Design review of the part built by this model. Coordinates are the model's own, in mm. Face numbers are marked on the shaded views. A direction names the side the tool comes from. Coordinates: 2 decimals unless noted, no trailing zeros. Loops run counter-clockwise (first coordinate to the right, second up) from the corner with the lowest first, then second, coordinate; pieces in that order, holes last.
Q1. Add section A-A on z = -67.5. Give the boundary of the cut face in (x, y) (3 decimals).
Q2. Wall thickness on probe 1 along X at (y, z) = (1.05, -67.5); probe 2 along Z at (x, y) = (-110, 2.7); probe 3 along X at (y, z) = (6, 0): over which ranges is each line inside the solid? List them lowest first.
Q3. Machinability: for the marked faces 1, 2, 3, 4 and 5, which of the approach directions +Z, -Z, +X, -X, +Y, -Y give a long, thin tool a straight path to every point of the face, cutting with its end or side? Answer none if there is none.
Q4. Add section C-C on y = 79. Give the boundary of the cut face in (x, z), and give its area (3 significant figures).
Q5. Add section B-B on x = -76. Give the boundary of the cut face in (y, z), and give its area (3 significant figures).
Q6. Add section D-D on z = -42. Give the boundary of the cut face in (x, y).
Q7. Draft analysis for pull direction X (two halves, no side actions). For the marked faces 6, 7, 8 and 9, state which applies: released by +X, released by -X, zero draft, split by the parting line, or undercut.
Q8. For P1, Ø5, axis at y = 19.5, z = 70, coming from the -X side; P2, Ø3, axis at y = 30, z = -65.5, coming from the -X side; P3, Ø4.5, axis at x = -113, z = -70.5, coming from the +Y side, all flat-tipped, find the tip position at first contact; note any pin that passes through.
```python
from build123d import *

# Parameters (mm, degrees)
SZKIC1_W                        = 200
SZKIC1_H                        = 200
DODANIE_WYCI_GNI_CIE1_DEPTH     = 30
WYTNIJ_WYCI_GNI_CIE1_DEPTH      = 145.568322948
WYTNIJ_WYCI_GNI_CIE1_DEPTH_BACK = 145.568322948
SZKIC2_W                        = 80
SZKIC2_H                        = 16
WYTNIJ_WYCI_GNI_CIE2_DEPTH      = 145.568322948
WYTNIJ_WYCI_GNI_CIE2_DEPTH_BACK = 145.568322948
SZKIC3_R                        = 20
SZKIC4_W                        = 28
SZKIC4_H                        = 16
DODANIE_WYCI_GNI_CIE2_DEPTH     = 9
DODANIE_WYCI_GNI_CIE3_START     = 30
SZKIC5_W                        = 50
SZKIC5_H                        = 50
DODANIE_WYCI_GNI_CIE3_DEPTH     = 40
DODANIE_WYCI_GNI_CIE4_START     = 70
SZKIC6_W                        = 151.215135745
SZKIC6_H                        = 50
SZKIC6_R                        = 9.5
DODANIE_WYCI_GNI_CIE4_DEPTH     = 5
DODANIE_WYCI_GNI_CIE5_START     = 75
SZKIC7_W                        = 151.215135745
SZKIC7_H                        = 50
SZKIC7_R                        = 15
DODANIE_WYCI_GNI_CIE5_DEPTH     = 15
DODANIE_WYCI_GNI_CIE6_START     = 60
DODANIE_WYCI_GNI_CIE6_DEPTH     = 25
WYTNIJ_WYCI_GNI_CIE3_DEPTH      = 181.277563773
WYTNIJ_WYCI_GNI_CIE4_START      = 5
WYTNIJ_WYCI_GNI_CIE4_DEPTH      = 176.277563773
SZYK_LINIOWY1_OUTLINE_R         = 7.5
SZYK_LINIOWY1_OUTLINE_R_2       = 2.75
SZYK_LINIOWY1_DEPTH             = 5
SZYK_LINIOWY1_2_OUTLINE_W       = 20
SZYK_LINIOWY1_2_OUTLINE_H       = 25
SZYK_LINIOWY1_2_OUTLINE_R       = 7.5
SZYK_LINIOWY1_2_DEPTH           = 30
SZYK_START                      = -113
SZYK_LINIOWY1_3_OUTLINE_W       = 35
SZYK_LINIOWY1_3_OUTLINE_H       = 25
SZYK_LINIOWY1_3_DEPTH           = 16.172267629
ZAOKR_GLENIE1_R                 = 20
SFAZOWANIE1_SIZE                = 10
SZKIC10_R                       = 2.6
WYTNIJ_WYCI_GNI_CIE5_DEPTH      = 176.957381204
WYTNIJ_WYCI_GNI_CIE6_DEPTH      = 181.277563773
WYTNIJ_WYCI_GNI_CIE6_DEPTH_BACK = 5
SZKIC11_R                       = 6


with BuildPart() as part:
    # Szkic1 → Dodanie-wyciągnięcie1 (new body)
    with BuildSketch(Plane(origin=(0, 0, 0), x_dir=(1, 0, 0), z_dir=(0, 1, 0))):
        Rectangle(SZKIC1_W, SZKIC1_H)
    extrude(amount=DODANIE_WYCI_GNI_CIE1_DEPTH)

    # Szkic2 → Wytnij-wyciągnięcie1 (cut, two sides: drawn at the far end of the back side and taken through both)
    with BuildSketch(Plane(origin=(0, 0, 0), x_dir=(1, 0, 0), z_dir=(0, 1, 0)).offset(-WYTNIJ_WYCI_GNI_CIE1_DEPTH_BACK)):
        Rectangle(SZKIC2_W, SZKIC2_H)
    extrude(amount=WYTNIJ_WYCI_GNI_CIE1_DEPTH + WYTNIJ_WYCI_GNI_CIE1_DEPTH_BACK, mode=Mode.SUBTRACT)

    # Szkic3 → Wytnij-wyciągnięcie2 (cut, two sides: drawn at the far end of the back side and taken through both)
    with BuildSketch(Plane(origin=(0, 0, 0), x_dir=(1, 0, 0), z_dir=(0, 1, 0)).offset(-WYTNIJ_WYCI_GNI_CIE2_DEPTH_BACK)):
        with Locations((33.228865647, 0)):
            Circle(SZKIC3_R)
    extrude(amount=WYTNIJ_WYCI_GNI_CIE2_DEPTH + WYTNIJ_WYCI_GNI_CIE2_DEPTH_BACK, mode=Mode.SUBTRACT)

    # Szkic4 → Dodanie-wyciągnięcie2 (add)
    with BuildSketch(Plane(origin=(0, 0, 0), x_dir=(1, 0, 0), z_dir=(0, 1, 0))):
        with Locations((-26, 0)):
            Rectangle(SZKIC4_W, SZKIC4_H)
    extrude(amount=DODANIE_WYCI_GNI_CIE2_DEPTH)

    # Szkic5 → Dodanie-wyciągnięcie3 (add)
    with BuildSketch(Plane(origin=(0, 0, 0), x_dir=(1, 0, 0), z_dir=(0, 1, 0)).offset(DODANIE_WYCI_GNI_CIE3_START)):
        with Locations((-70, 0)):
            Rectangle(SZKIC5_W, SZKIC5_H)
    extrude(amount=DODANIE_WYCI_GNI_CIE3_DEPTH)

    # Szkic6 → Dodanie-wyciągnięcie4 (add)
    with BuildSketch(Plane(origin=(0, 0, 0), x_dir=(1, 0, 0), z_dir=(0, 1, 0)).offset(DODANIE_WYCI_GNI_CIE4_START)):
        with Locations((-19.392432127, 0)):
            Rectangle(SZKIC6_W, SZKIC6_H)
        with Locations(Location((33.228865647, 0, 0), (0, 0, 90))):
            Circle(SZKIC6_R, mode=Mode.SUBTRACT)
    extrude(amount=DODANIE_WYCI_GNI_CIE4_DEPTH)

    # Szkic7 → Dodanie-wyciągnięcie5 (add)
    with BuildSketch(Plane(origin=(0, 0, 0), x_dir=(1, 0, 0), z_dir=(0, 1, 0)).offset(DODANIE_WYCI_GNI_CIE5_START)):
        with Locations((-19.392432127, 0)):
            Rectangle(SZKIC7_W, SZKIC7_H)
        with Locations(Location((33.228865647, 0, 0), (0, 0, 270))):
            Circle(SZKIC7_R, mode=Mode.SUBTRACT)
    extrude(amount=DODANIE_WYCI_GNI_CIE5_DEPTH)

    # Szkic8 → Dodanie-wyciągnięcie6 (add)
    with BuildSketch(Plane.XY.offset(DODANIE_WYCI_GNI_CIE6_START)):
        Polygon((-100, 0), (-120, 0), (-120, 5), (-100, 30), align=None)
    dodanie_wyci_gni_cie6 = extrude(amount=DODANIE_WYCI_GNI_CIE6_DEPTH)

    # Szkic9 → Wytnij-wyciągnięcie3 (cut, symmetric)
    with BuildSketch(Plane(origin=(0, 0, 0), x_dir=(1, 0, 0), z_dir=(0, 1, 0))):
        with BuildLine():
            ThreePointArc((-107.25, -72.5), (-107.5214161, -71.308730991), (-108.282088619, -70.352610774))
            Line((-108.282088619, -70.352610774), (-111.717911381, -74.647389226))
            ThreePointArc((-111.717911381, -74.647389226), (-108.808730991, -74.9785839), (-107.25, -72.5))
        make_face()
        with BuildLine():
            Line((-111.717911381, -74.647389226), (-108.282088619, -70.352610774))
            ThreePointArc((-108.282088619, -70.352610774), (-112.147389226, -70.782088619), (-111.717911381, -74.647389226))
        make_face()
    wytnij_wyci_gni_cie3 = extrude(amount=WYTNIJ_WYCI_GNI_CIE3_DEPTH, both=True, mode=Mode.SUBTRACT)

    # Szkic9<3> → Wytnij-wyciągnięcie4 (cut, through all)
    with BuildSketch(Plane(origin=(0, 0, 0), x_dir=(1, 0, 0), z_dir=(0, 1, 0)).offset(WYTNIJ_WYCI_GNI_CIE4_START)):
        with BuildLine():
            ThreePointArc((-102.5, -72.5), (-103.240225728, -69.251084521), (-105.314787143, -66.643483929))
            Line((-105.314787143, -66.643483929), (-108.282088619, -70.352610774))
            ThreePointArc((-108.282088619, -70.352610774), (-107.5214161, -71.308730991), (-107.25, -72.5))
            ThreePointArc((-107.25, -72.5), (-108.808730991, -74.9785839), (-111.717911381, -74.647389226))
            Line((-111.717911381, -74.647389226), (-114.685212857, -78.356516071))
            ThreePointArc((-114.685212857, -78.356516071), (-106.751084521, -79.259774272), (-102.5, -72.5))
        make_face()
        with BuildLine():
            Line((-108.282088619, -70.352610774), (-105.314787143, -66.643483929))
            ThreePointArc((-105.314787143, -66.643483929), (-115.856516071, -67.814787143), (-114.685212857, -78.356516071))
            Line((-114.685212857, -78.356516071), (-111.717911381, -74.647389226))
            ThreePointArc((-111.717911381, -74.647389226), (-112.147389226, -70.782088619), (-108.282088619, -70.352610774))
        make_face()
    wytnij_wyci_gni_cie4 = extrude(amount=WYTNIJ_WYCI_GNI_CIE4_DEPTH, mode=Mode.SUBTRACT)



with BuildPart() as body_2:
    # Szyk liniowy1: read off the stored shape, not the designer's step
    # Szyk liniowy1 outline → Szyk liniowy1 (new body)
    with BuildSketch(Plane(origin=(0, 0, 0), x_dir=(1, 0, 0), z_dir=(0, 1, 0))):
        with Locations((-110, 67.5)):
            Circle(SZYK_LINIOWY1_OUTLINE_R)
        with Locations((-110, 67.5)):
            Circle(SZYK_LINIOWY1_OUTLINE_R_2, mode=Mode.SUBTRACT)
    szyk_liniowy1 = extrude(amount=SZYK_LINIOWY1_DEPTH)


with BuildPart() as part_1:
    add(part.part)

    add(body_2.part)  # Szyk liniowy1 2 merges body 2
    # Szyk liniowy1 2 outline → Szyk liniowy1 2 (add)
    with BuildSketch(Plane(origin=(0, 0, 0), x_dir=(1, 0, 0), z_dir=(0, 1, 0))):
        with Locations((-110, 67.5)):
            Rectangle(SZYK_LINIOWY1_2_OUTLINE_W, SZYK_LINIOWY1_2_OUTLINE_H)
        with Locations((-110, 67.5)):
            Circle(SZYK_LINIOWY1_2_OUTLINE_R, mode=Mode.SUBTRACT)
    szyk_liniowy1_2 = extrude(amount=SZYK_LINIOWY1_2_DEPTH)

    # Szyk liniowy1 3 outline → Szyk liniowy1 3 (cut)
    with BuildSketch(Plane(origin=(0, 0, 0), x_dir=(0.6246950475544242, 0.7808688094430304, 0), z_dir=(0.7808688094430304, -0.6246950475544242, 0)).offset(SZYK_START)):
        with Locations((-55.5, -67.5)):
            Rectangle(SZYK_LINIOWY1_3_OUTLINE_W, SZYK_LINIOWY1_3_OUTLINE_H)
    szyk_liniowy1_3 = extrude(amount=SZYK_LINIOWY1_3_DEPTH, mode=Mode.SUBTRACT)

    # Lustro1: Dodanie-wyciągnięcie6, Wytnij-wyciągnięcie3, Wytnij-wyciągnięcie4, Szyk liniowy1, Szyk liniowy1 2, Szyk liniowy1 3 across plane
    add(dodanie_wyci_gni_cie6.mirror(Plane(origin=(0, 0, 0), x_dir=(0, 0, 1), z_dir=(1, 0, 0))))
    add(wytnij_wyci_gni_cie3.mirror(Plane(origin=(0, 0, 0), x_dir=(0, 0, 1), z_dir=(1, 0, 0))), mode=Mode.SUBTRACT)
    add(wytnij_wyci_gni_cie4.mirror(Plane(origin=(0, 0, 0), x_dir=(0, 0, 1), z_dir=(1, 0, 0))), mode=Mode.SUBTRACT)
    add(szyk_liniowy1.mirror(Plane(origin=(0, 0, 0), x_dir=(0, 0, 1), z_dir=(1, 0, 0))))
    add(szyk_liniowy1_2.mirror(Plane(origin=(0, 0, 0), x_dir=(0, 0, 1), z_dir=(1, 0, 0))))
    add(szyk_liniowy1_3.mirror(Plane(origin=(0, 0, 0), x_dir=(0, 0, 1), z_dir=(1, 0, 0))), mode=Mode.SUBTRACT)

    # Zaokrąglenie1
    # the kernel refuses this fillet: 20 mm, written as the material it takes off along each edge
    with BuildSketch(Plane(origin=(-100, -48.412291828, 100), x_dir=(1, 0, 0), z_dir=(0, 1, 0))) as zaokr_glenie1_piece_1:
        with BuildLine():
            CenterArc((19.364916731, 20), ZAOKR_GLENIE1_R, 194.477512186, 75.522487814)
            Line((0, 15), (-0.387298335, 14.9))
            ThreePointArc((-0.387298335, 14.9), (-0.4, 7.5), (-0.4, 0))
            Line((-0.4, 0), (0, -0.4))
            Line((0, -0.4), (19.364916731, -0.4))
            Line((19.364916731, -0.4), (19.364916731, 0))
        make_face()
    extrude(amount=126.824583655, mode=Mode.SUBTRACT)
    with BuildSketch(Plane(origin=(-100, -50, -100), x_dir=(0, 0, 1), z_dir=(0, 1, 0)), Plane(origin=(100, -50, -100), x_dir=(-1, 0, 0), z_dir=(0, 1, 0))) as zaokr_glenie1_piece_2:
        with BuildLine():
            CenterArc((ZAOKR_GLENIE1_R, ZAOKR_GLENIE1_R), ZAOKR_GLENIE1_R, 180, 90)
            Line((0, ZAOKR_GLENIE1_R), (-ZAOKR_GLENIE1_R * 0.02, ZAOKR_GLENIE1_R))
            Line((-ZAOKR_GLENIE1_R * 0.02, ZAOKR_GLENIE1_R), (-ZAOKR_GLENIE1_R * 0.02, -ZAOKR_GLENIE1_R * 0.02))
            Line((-ZAOKR_GLENIE1_R * 0.02, -ZAOKR_GLENIE1_R * 0.02), (ZAOKR_GLENIE1_R, -ZAOKR_GLENIE1_R * 0.02))
            Line((ZAOKR_GLENIE1_R, -ZAOKR_GLENIE1_R * 0.02), (ZAOKR_GLENIE1_R, 0))
        make_face()
    extrude(amount=130, mode=Mode.SUBTRACT)
    with BuildSketch(Plane(origin=(100, -48.412291828, 100), x_dir=(-1, 0, 0), z_dir=(0, 1, 0))) as zaokr_glenie1_piece_3:
        with BuildLine():
            CenterArc((19.364916731, -20), ZAOKR_GLENIE1_R, 90, 75.522487814)
            Line((0, -15), (-0.387298335, -14.9))
            ThreePointArc((-0.387298335, -14.9), (-0.4, -7.5), (-0.4, 0))
            Line((-0.4, 0), (0, 0.4))
            Line((0, 0.4), (19.364916731, 0.4))
            Line((19.364916731, 0.4), (19.364916731, 0))
        make_face()
    extrude(amount=126.824583655, mode=Mode.SUBTRACT)

    # Sfazowanie1
    sfazowanie1_edges = [part_1.edges().sort_by_distance(p)[0] for p in [
        (-45, 70, 0),
    ]]
    chamfer(sfazowanie1_edges, length=SFAZOWANIE1_SIZE)

    # Szkic10 → Wytnij-wyciągnięcie5 (cut, through all)
    with BuildSketch(Plane(origin=(0, 9, 0), x_dir=(1, 0, 0), z_dir=(0, 1, 0))):
        with Locations(Location((-35, 0, 0), (0, 0, 270))):
            Circle(SZKIC10_R)
        with Locations(Location((-20, 0, 0), (0, 0, 270))):
            Circle(SZKIC10_R)
    extrude(amount=-WYTNIJ_WYCI_GNI_CIE5_DEPTH, mode=Mode.SUBTRACT)

    # Szkic11 → Wytnij-wyciągnięcie6 (cut, two sides: drawn at the far end of the back side and taken through both)
    with BuildSketch(Plane(origin=(0, 0, 0), x_dir=(-1, 0, 0), z_dir=(0, -1, 0)).offset(-WYTNIJ_WYCI_GNI_CIE6_DEPTH_BACK)):
        with Locations(Location((20, 0, 0), (0, 0, 270))):
            Circle(SZKIC11_R)
        with Locations(Location((35, 0, 0), (0, 0, 270))):
            Circle(SZKIC11_R)
    extrude(amount=WYTNIJ_WYCI_GNI_CIE6_DEPTH + WYTNIJ_WYCI_GNI_CIE6_DEPTH_BACK, mode=Mode.SUBTRACT)


solid = part_1.part
```
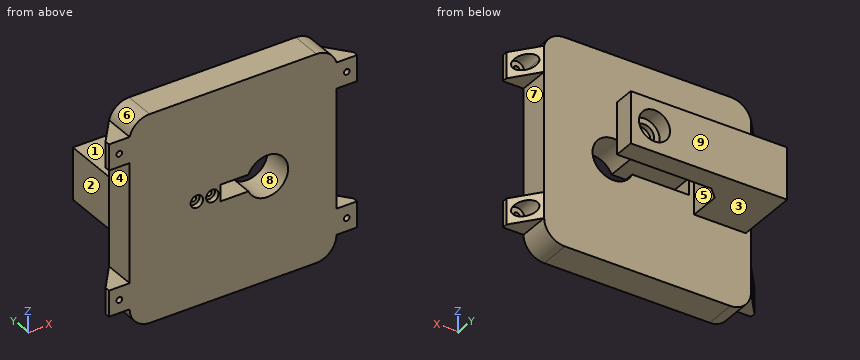
Entries:
1. outline: (-120, 0) - (-112.75, 0) - (-112.75, 5) - (-117.5, 5) - (-117.5, 8.125) - (-120, 5) - close; (-107.25, 0) - (107.25, 0) - (107.25, 5) - (102.5, 5) - (102.5, 26.875) - (100, 30) - (-100, 30) - (-102.5, 26.875) - (-102.5, 5) - (-107.25, 5) - close; (112.75, 0) - (120, 0) - (120, 5) - (117.5, 8.125) - (117.5, 5) - (112.75, 5) - close
2. probe 1: x = -120 to -112.75, -107.25 to 107.25, 112.75 to 120
2. probe 2: z = -80 to -70.25, -64.75 to -55, 60 to 69.75, 75.25 to 85
2. probe 3: x = -100 to -37.6, -32.4 to -22.6, -17.4 to -12, 53.23 to 100
3. face 1: +Z, +X, -X, +Y
3. face 2: +Z, -Z, -X, +Y
3. face 3: -Z, +X, -X, +Y
3. face 4: -X, +Y, -Y
3. face 5: +Z, -Z, +X
4. outline: (-95, -25) - (56.22, -25) - (56.22, 25) - (-95, 25) - close; hole circle Ø30 at (33.23, 0)
4. area: 6,850 mm2
5. outline: (0, -100) - (30, -100) - (30, -25) - (90, -25) - (90, 25) - (30, 25) - (30, 100) - (0, 100) - close
5. area: 9,000 mm2
6. outline: (-100, 0) - (100, 0) - (100, 30) - (-100, 30) - close
7. face 6: released by -X
7. face 7: released by +X
7. face 8: undercut
7. face 9: zero draft
8. P1: stops at x = -104.41
8. P2: stops at x = -101.2
8. P3: stops at y = 5
